from build123d import *

# Parameters (mm, degrees)
SKETCH_W      = 100
SKETCH_H      = 100
PAD_DEPTH     = 10
SKETCH001_R   = 50
SKETCH001_R_2 = 40
SKETCH001_W   = 50
SKETCH001_H   = 50
POCKET_DEPTH  = 5


with BuildPart() as part:
    # Sketch → Pad (new body)
    with BuildSketch(Plane.XY):
        Rectangle(SKETCH_W, SKETCH_H)
    extrude(amount=PAD_DEPTH)

    # Sketch001 (on Face6 of Pad) → Pocket (cut)
    with BuildSketch(Plane.XY.offset(10)):
        with Locations((65, 0)):
            Circle(SKETCH001_R)
        with Locations((65, 0)):
            Circle(SKETCH001_R_2, mode=Mode.SUBTRACT)
        with Locations((-30, 0)):
            Rectangle(SKETCH001_W, SKETCH001_H)
    extrude(amount=-POCKET_DEPTH, mode=Mode.SUBTRACT)


solid = part.part
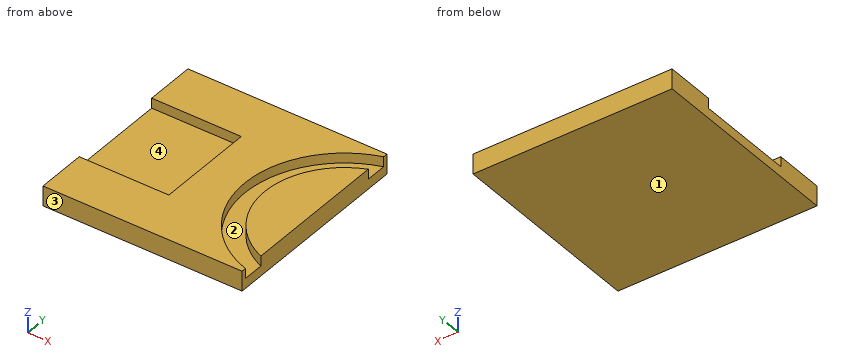
Build history of the part. All positions in model axes, mm. Face numbers are marked on the shaded views. Round coordinates to 2 decimals unless told otherwise and drop trailing zeros. Order: outer loops, then holes, each group sorted by start corner. A loop starts at its lowest first (then second) coordinate and runs counter-clockwise, first axis right, second up. Notation, with made-up numbers: M 58,-21.75 L 100,-21.75 A13 ccw 100,-0.75 Z; hole C -9,-24 d10. An arc over 180 degrees is marked long. Use CSV: the item, a comma, the result in double quotes. Start each with the question number.
(1) Cut at D-D on x = 20.5. List the corners of the cut face in (y, z).
(2) Mould opens along Y. For the marked faces 1, 2, 3 and 4 say: +Y half, -Y half, draft (parallel to the pull), parting line (faces both ways), or undercut.
(3) Flat gauge pins, fed straight in: P1, Ø4, axis at x = -19.5, y = -20, coming from the -Z side; P2, Ø1.5, axis at y = 14, z = 6.5, coming from the -X side. Where does each tip first touch, or does it go through?
(4) Drill centre lines: probe 1 along Y at (x, z) = (-36.5, 8.5); probe 2 along Z at (x, y) = (-13.5, 24); probe 3 along X at (y, z) = (19.5, 7.75). Where is each one in solid material? Low to high.
(5) Cut at A-A on z = 8.75. List the corners of the cut face in (x, y), then the cut area to 3 significant figures.
(6) Cut at C-C on y = -12. List the corners of the cut face in (x, z).
(7) Cut at B-B on x = -43. List the corners of the cut face in (y, z).
Findings:
1,outline,"M -50,0 L 50,0 L 50,10 L 22.8,10 L 22.8,5 L -22.8,5 L -22.8,10 L -50,10 Z"
2,face 1,"draft"
2,face 2,"undercut"
2,face 3,"-Y half"
2,face 4,"undercut"
3,P1,"stops at z = 0"
3,P2,"stops at x = -5"
4,probe 1,"y = -50 to -25, 25 to 50"
4,probe 2,"z = 0 to 5"
4,probe 3,"x = -5 to 18.96, 30.08 to 50"
5,outline,"M -50,-50 L 50,-50 L 50,-47.7 A50 cw 50,47.7 L 50,50 L -50,50 L -50,25 L -5,25 L -5,-25 L -50,-25 Z; M 50,-37.08 L 50,37.08 A40 ccw Z"
5,area,"6,640 mm^2"
6,outline,"M -50,0 L 50,0 L 50,10 L 26.84,10 L 26.84,5 L 16.46,5 L 16.46,10 L -5,10 L -5,5 L -50,5 Z"
7,outline,"M -50,0 L 50,0 L 50,10 L 25,10 L 25,5 L -25,5 L -25,10 L -50,10 Z"
